Could you check a few things on this model? Use its own coordinates, in mm. Face numbers are marked on the shaded views. A direction names the side the tool comes from. Give positions to 0.01 mm unless a question says otherwise; leave off trailing zeros. Order: outer loops, then holes, each group sorted by start corner. A loop starts at its lowest first (then second) coordinate and runs counter-clockwise, first axis right, second up. Notation, with made-up numbers: (-12.5, 37) -> (-1.5, 37) arc R9 ccw to (-1.5, 51) -> close; hole circle Ø1 at (2, 12.25). An arc over 180 degrees is marked (long way). Answer as CSV lines item,"result". Start each with the question number.
(1) I want a section at C-C (y = 7.5). Please give me the cut outline in (x, z), plus the area to 3 significant figures.
(2) We'd pull the mould along X, two halves only. Please class the marked faces 1, 2 and 3: released by +X, released by -X, zero draft, split by the parting line, or undercut.
(3) I want a section at A-A (z = 2.5). Please give me the cut outline in (x, y).
(4) Will these pins go through, and if not, where does the flat tip stop? pin 1 Ø1.5 at (y, z) = (7, 1.5) entering from -X; pin 2 Ø1.5 at (y, z) = (6.5, 0.5) entering from -X; pin 3 Ø1 at (x, y) = (1.5, 4.5) entering from -Z.
(5) On a 3-axis mill with a long thin cutter (end or side, diameter ignored), from which of +Z, -Z, +X, -X, +Y, -Y can I reach the whole of each face in a straight line? I mean the marked faces 4 and 5. Say none if no direction works.
(6) I want a section at D-D (z = 3.2). Please give me the cut outline in (x, y), plus the area to 3 significant figures.
(7) I need wall thicknesses on L1, parallel to X at y = 6.5, z = 3.2; L2, parallel to X at y = 6.5, z = 2.1; L3, parallel to Z at x = 3.5, y = 2. Which ranges of each line are inside material? Lowest first, please.
(8) I want a section at B-B (x = 2.5). Please give me the cut outline in (y, z).
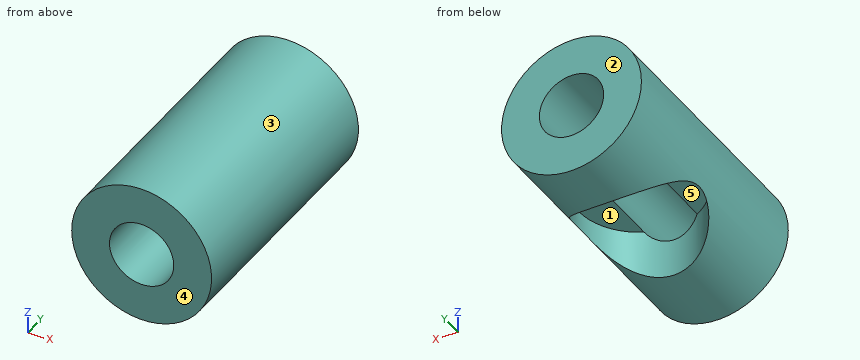
Autodesk Inventor part; units mm, degrees
ref_plane "screwMaxDist" through (2.5, 0, 1.85) normal (0, 0, 1) x (1, 0, 0)
ref_plane "YZ Plane" through (0, 0, 0) normal (1, 0, 0) x (0, 1, 0)
ref_plane "XZ Plane" through (0, 0, 0) normal (0, 1, 0) x (-1, 0, 0)
sketch "Sketch1" plane through (0, 0, 0) normal (0, 1, 0) x (-1, 0, 0)
  circle A0 centre (-2.5, 2.5) radius 1.15
  circle A1 centre (-2.5, 2.5) radius 2.5
  line L0 (0, 0) -> (-7.3028, 0) construction
  line L1 (0, 0) -> (0, 4.3038) construction
  dimension "d0" = 2.3
  dimension "d1" = 5
extrude "Extrusion1" add sketch "Sketch1" along normal blind 9
ref_plane "Work Plane1" through (2.5, 0, 1.35) normal (0, 0, 1) x (1, 0, 0)
ref_plane "screwMaxDist" through (2.5, 0, 1.85) normal (0, 0, 1) x (1, 0, 0)
sketch "Sketch2" plane through (0, 0, 0) normal (0, 0, 1) x (1, 0, 0)
  line L0 (5, 9) -> (0, 9)
  circle A0 centre (2.5, 4.85) radius 2.15
  line L1 (5, 9) -> (0, 9)
  line L2 (5, 0) -> (0, 0)
  line L3 (0, 0) -> (0, 9)
  line L4 (0, 7) -> (5, 7)
  line L5 (5, 0) -> (5, 9)
  dimension "d5" = 4.3
  dimension "d15" = 2
  dimension "d16" = 2.5
  dimension "d17" = 2.5
extrude "Extrusion2" cut sketch "Sketch2" along normal up to surface (1.85 mm away) contours A0
equation "\"d16\" = d17"
properties part number "motor_shaft_adapter" material "ABS Plastic"
Final values:
1,outline,"circle Ø5 at (2.5, 2.5); hole circle Ø2.3 at (2.5, 2.5)"
1,area,"15.5 mm²"
2,face 1,"undercut"
2,face 2,"zero draft"
2,face 3,"split by the parting line"
3,outline,"(0, 0) -> (1.35, 0) -> (1.35, 9) -> (0, 9) -> close; (3.65, 0) -> (5, 0) -> (5, 9) -> (3.65, 9) -> close"
4,pin 1,"x = 0.01"
4,pin 2,"x = 0.33"
4,pin 3,"z = 1.85"
5,face 4,"+Z, -Z, +X, -X, -Y"
5,face 5,"-Z"
6,outline,"(0.1, 0) -> (1.59, 0) -> (1.59, 9) -> (0.1, 9) -> close; (3.41, 0) -> (4.9, 0) -> (4.9, 9) -> (3.41, 9) -> close"
6,area,"26.8 mm²"
7,L1,"0.1 to 1.59, 3.41 to 4.9"
7,L2,"0.03 to 1.42, 3.58 to 4.97"
7,L3,"0.21 to 1.93, 3.07 to 4.79"
8,outline,"(0, 0) -> (2.7, 0) -> (2.7, 1.35) -> (0, 1.35) -> close; (0, 3.65) -> (9, 3.65) -> (9, 5) -> (0, 5) -> close; (7, 0) -> (9, 0) -> (9, 1.35) -> (7, 1.35) -> close"
